from build123d import *

# Parameters (mm, degrees)
ESQUISSE1_W        = 2
ESQUISSE1_H        = 31
BOSS_EXTRU_1_DEPTH = 10
CONG_1_R           = 1


with BuildPart() as part:
    # Esquisse1 → Boss.-Extru.1 (new body)
    with BuildSketch(Plane.XY):
        Polygon((10.551419921, 0), (10.551419921, 1.805779869), (6.81110646, 3.223544029), (2.31110646, 3.223544029), (-1.448580079, 1.857982926), (-1.448580079, 0), (2.051419921, 0), (2.051419921, -32.5), (7.051419921, -32.5), (7.051419921, 0), align=None)
        with Locations((4.551419921, -15.5)):
            Rectangle(ESQUISSE1_W, ESQUISSE1_H, mode=Mode.SUBTRACT)
    extrude(amount=BOSS_EXTRU_1_DEPTH)

    # Congé1
    cong_1_edges = [part.edges().sort_by_distance(p)[0] for p in [
        (-1.448580079, 0, 5),
        (-1.448580079, 1.857982926, 5),
        (2.31110646, 3.223544029, 5),
        (6.81110646, 3.223544029, 5),
        (10.551419921, 1.805779869, 5),
        (10.551419921, 0, 5),
        (7.051419921, -32.5, 5),
        (2.051419921, -32.5, 5),
    ]]
    fillet(cong_1_edges, radius=CONG_1_R)


solid = part.part
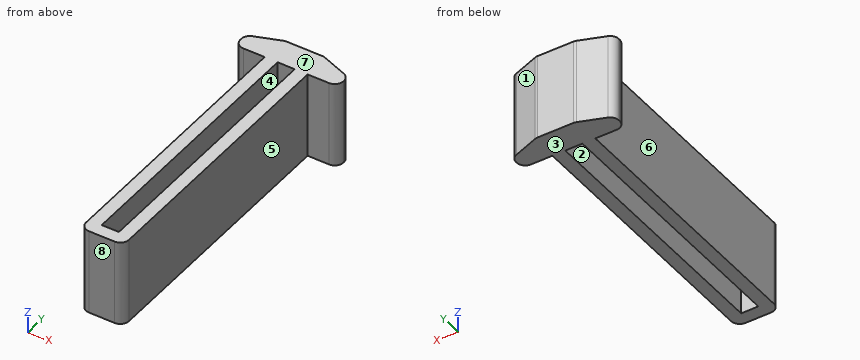
Work out the finished part from the listing and answer in its coordinate system (mm). Face numbers are marked on the shaded views. A direction names the side the tool comes from. Give positions to 0.01 mm unless a question says otherwise; leave off trailing zeros. Loops run counter-clockwise (first coordinate to the right, second up) from the corner with the lowest first, then second, coordinate; pieces in that order, holes last. Notation, with made-up numbers: (8.25, 18.5) -> (18.25, 18.5) arc R18 cw to (18.25, 35.5) -> close; hole circle Ø7 at (61.25, 75). An arc over 180 degrees is marked (long way). Use a Markdown table: item, result. Add a question column.
1) Consider line 1 along X through (y, z) = (-9, 4.25); line 2 along Y through (x, z) = (5, 9); line 3 along Y through (x, z) = (1.5, 2.5). Determine where each line is inside the solid, lowest interval first.
2) Each of these flat-tipped pins is pushed along its axis until it touches: P1, Ø2, axis at x = 8.5, z = 4, coming from the -Y side; P2, Ø2, axis at y = -21.5, z = 4, coming from the +X side. Where does it stop, or does it pass through?
3) The part is cut by section A-A, the plane y = -20. Determine the outline of the cut face in (x, z), plus the area to 3 significant figures.
4) The part is cut by section C-C, the plane x = 8. Determine the outline of the cut face in (y, z).
5) Which of the six approach directions +Z, -Z, +X, -X, +Y, -Y give full straight-line access (tool end or side, diameter ignored) to the marked faces 4, 5, 6, 7 and 8?
6) The part is cut by section B-B, the plane z = 5.5. Determine the outline of the cut face in (x, y), plus the area to 3 significant figures.
7) The part is cut by section D-D, the plane x = 1.5. Determine the outline of the cut face in (y, z).
8) For a pull along X with two mould halves and no side action, classify the marked faces 1, 2 and 3 as +X half, -X half, draft (parallel to the pull), parting line (faces both ways), or undercut.
Reported:
| question | item | result |
|---|---|---|
| 1 | line 1 | x = 2.05 to 3.55, 5.55 to 7.05 |
| 1 | line 2 | y = -32.5 to -31, 0 to 3.22 |
| 1 | line 3 | y = 0 to 2.93 |
| 2 | P1 | stops at y = 0 |
| 2 | P2 | stops at x = 7.05 |
| 3 | outline | (2.05, 0) -> (3.55, 0) -> (3.55, 10) -> (2.05, 10) -> close; (5.55, 0) -> (7.05, 0) -> (7.05, 10) -> (5.55, 10) -> close |
| 3 | area | 30.0 mm^2 |
| 4 | outline | (0, 0) -> (2.77, 0) -> (2.77, 10) -> (0, 10) -> close |
| 5 | face 4 | +Z, -Z |
| 5 | face 5 | +Z, -Z, +X, -Y |
| 5 | face 6 | +Z, -Z, -X, -Y |
| 5 | face 7 | +Z, +X, -X, +Y, -Y |
| 5 | face 8 | +Z, -Z, +X, -X, -Y |
| 6 | outline | (-1.45, 1) arc R1 ccw to (-0.45, 0) -> (2.05, 0) -> (2.05, -31.5) arc R1 ccw to (3.05, -32.5) -> (6.05, -32.5) arc R1 ccw to (7.05, -31.5) -> (7.05, 0) -> (9.55, 0) arc R1 ccw to (10.55, 1) -> (10.55, 1.12) arc R1 ccw to (9.91, 2.05) -> (6.98, 3.16) arc R1 ccw to (6.63, 3.22) -> (2.49, 3.22) arc R1 ccw to (2.15, 3.16) -> (-0.79, 2.1) arc R1 ccw to (-1.45, 1.16) -> close; hole (3.55, -31) -> (5.55, -31) -> (5.55, 0) -> (3.55, 0) -> close |
| 6 | area | 133 mm^2 |
| 7 | outline | (0, 0) -> (2.93, 0) -> (2.93, 10) -> (0, 10) -> close |
| 8 | face 1 | +X half |
| 8 | face 2 | undercut |
| 8 | face 3 | draft |
